Job drawing, mm, ordinate dimensions from the low corner. One solid piece. A direction names the side the tool comes from. Round coordinates to 2 decimals unless told otherwise and drop trailing zeros. Order: outer loops, then holes, each group sorted by start corner. A loop starts at its lowest first (then second) coordinate and runs counter-clockwise, first axis right, second up. Notation, with made-up numbers: (65, 21.25) -> (92, 21.25) arc R22 ccw to (92, 35.25) -> close; hole circle Ø2 at (-36.5, 75.5). An arc over 180 degrees is marked (long way). Return JSON: item names as keys, results as strings. Group by question number.
Q1. Cut at B-B (x = 8). Write the cut outline in (y, z), then the cut area to 4 significant figures.
Q2. Which spindle directions (+Z, -Z, +X, -X, +Y, -Y) get a long thin tool onto all of the face, cutting with end or side? Do the marked faces 4, 5 and 6. Say none if no direction does.
Q3. Mould opens along Y. For the marked faces 1, 2 and 3 say: +Y half, -Y half, draft (parallel to the pull), parting line (faces both ways), or undercut.
Q4. Cut at D-D (y = 14.5). Write the cut outline in (x, z).
Q5. Flat gauge pins, fed straight in: pin 1 (2 mm diameter, centred on x = 5.5, z = 7.5, fed in from +Y); pin 2 (2.5 mm diameter, centred on y = 3.5, z = 8, fed in from -X); pin 3 (4 mm diameter, centred on x = 3, y = 12.5, fed in from +Z); pin 4 (1.5 mm diameter, centred on y = 3.5, z = 11.5, fed in from +X). Where does each tip first touch, or does it go through?
Q6. Cut at A-A (z = 8). Write the cut outline in (x, y).
Q7. Probe line 1 along Y through (x, z) = (2.5, 11); line 2 along X through (y, z) = (11.75, 8); line 3 along Z through (x, y) = (10.5, 13.25). List the from-to ranges inside material, lowest first.
Q8. Cut at C-C (y = 3.5). Write the cut outline in (x, z), then the cut area to 3 significant figures.
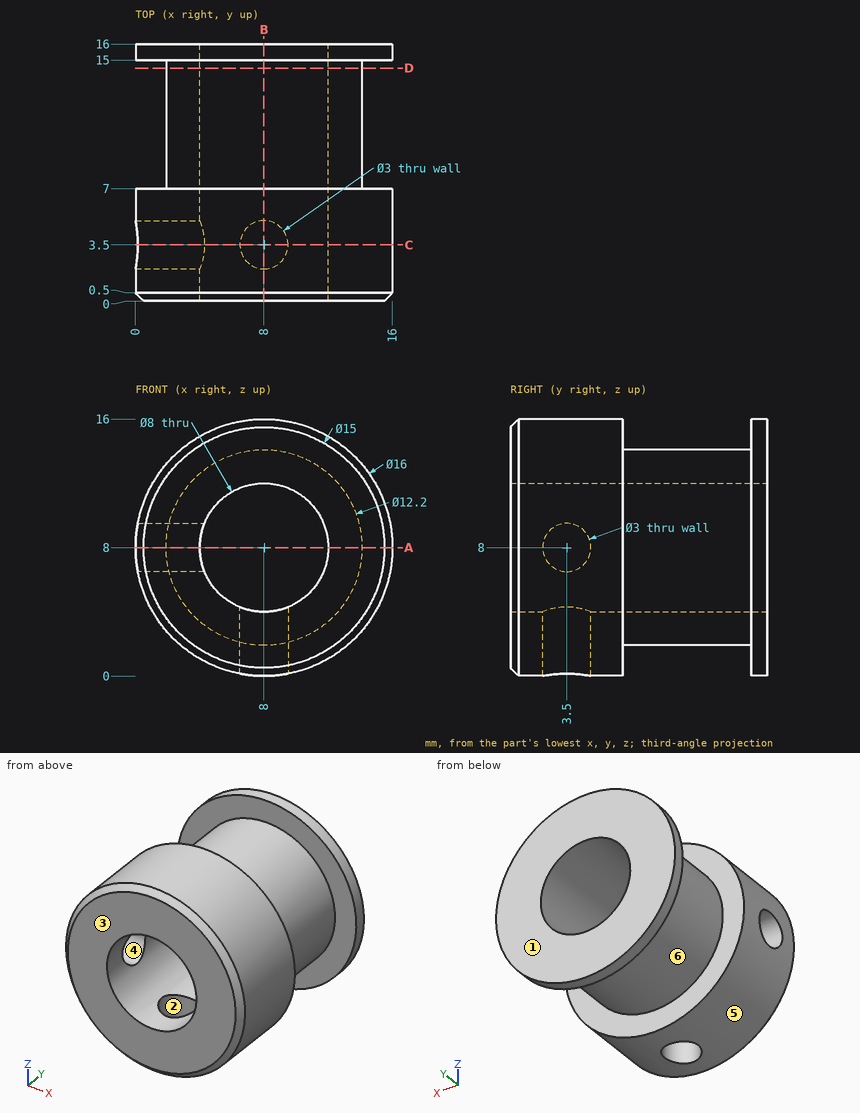
Solution:
{
 "1": {"outline": "(0, 0.5) -> (0.5, 0) -> (2, 0) -> (2, 4) -> (0, 4) -> close; (0, 12) -> (16, 12) -> (16, 16) -> (15, 16) -> (15, 14.1) -> (7, 14.1) -> (7, 16) -> (0.5, 16) -> (0, 15.5) -> close; (5, 0) -> (7, 0) -> (7, 1.9) -> (15, 1.9) -> (15, 0) -> (16, 0) -> (16, 4) -> (5, 4) -> close", "area": "85.35 mm²"},
 "2": {"face 4": "-X", "face 5": "+Y, -Y", "face 6": "none"},
 "3": {"face 1": "+Y half", "face 2": "undercut", "face 3": "-Y half"},
 "4": {"outline": "circle Ø12.2 at (8, 8); hole circle Ø8 at (8, 8)"},
 "5": {"pin 1": "passes through", "pin 2": "stops at x = 11.8", "pin 3": "stops at z = 13.31", "pin 4": "stops at x = 15.51"},
 "6": {"outline": "(0, 0.5) -> (0.5, 0) -> (4, 0) -> (4, 2) -> (0, 2) -> close; (0, 5) -> (4, 5) -> (4, 16) -> (0, 16) -> (0, 15) -> (1.9, 15) -> (1.9, 7) -> (0, 7) -> close; (12, 0) -> (15.5, 0) -> (16, 0.5) -> (16, 7) -> (14.1, 7) -> (14.1, 15) -> (16, 15) -> (16, 16) -> (12, 16) -> close"},
 "7": {"line 1": "y = 0 to 7, 15 to 16", "line 2": "x = 1.9 to 4, 12 to 14.1", "line 3": "z = 2.44 to 4.88, 11.12 to 13.56"},
 "8": {"outline": "(0.14, 6.5) arc R8 ccw to (6.5, 0.14) -> (6.5, 4.29) arc R4 cw to (4.29, 6.5) -> close; (0.14, 9.5) -> (4.29, 9.5) arc R4 cw (long way) to (9.5, 4.29) -> (9.5, 0.14) arc R8 ccw (long way) to start", "area": "127 mm²"}
}
